Geometry check sheet. Reference: the model listing, model coordinates, mm. A direction names the side the tool comes from. Give positions to 0.01 mm unless a question says otherwise; leave off trailing zeros. Loops run counter-clockwise (first coordinate to the right, second up) from the corner with the lowest first, then second, coordinate; pieces in that order, holes last. Notation, with made-up numbers: (18, -21) -> (37, -21) arc R30 ccw to (37, 8) -> close; hole circle Ø9 at (-37.75, 49). An arc over 180 degrees is marked (long way). Write each question's results on one line, items separated by ' | '. Start each with the question number.
1) Sectioned sample at C-C on z = -4.15. Record the cut outline in (x, y).
2) Sectioned sample at A-A on y = 0. Record the cut outline in (x, z).
3) Scan lines: line 1 (Y direction, x = 0, z = -1.9); line 2 (Z direction, x = 5, y = 0.5); line 3 (Y direction, x = -2, z = -2.35). Record each from-to range of solid material in increasing order. Write a range as from..to.
4) Set-up check for faces 1 (the face through (5.96, -1.88, -0.51)), 2 (the face through (-1, 5, -1)): record each of +Z, -Z, +X, -X, +Y, -Y from which the full face is reachable in a straight line by a thin tool's end or side.
5) Depth check by flat-ended pin: pin 1 (2 mm diameter, centred on x = 2.5, z = -5, fed in from -Y); pin 2 (3 mm diameter, centred on y = 4, z = -1.5, fed in from -X); pin 3 (5.5 mm diameter, centred on x = 0, y = 0, fed in from +Z). Enter the tip coordinate at first touch or a pass-through.
6) Sectioned sample at D-D on x = 5.75. Record the cut outline in (y, z).
```python
from build123d import *


# Read off the part's stored shape, not the designer's step: Оболочка1
with BuildPart() as part:
    # Эскиз1 → Повернуть1 (revolve)
    with BuildSketch(Plane(origin=(0, 0, 0), x_dir=(1, 0, 0), z_dir=(0, 1, 0))):
        with BuildLine():
            Line((0, 6), (0, 1))
            Line((0, 1), (3.872983346, 1))
            ThreePointArc((3.872983346, 1), (3.968118785, 1.49598283), (4, 2))
            ThreePointArc((4, 2), (2.828427125, 4.828427125), (0, 6))
        make_face()
        with BuildLine():
            Line((3.872983346, 1), (0, 1))
            Line((0, 1), (0, 0))
            Line((0, 0), (3.464101615, 0))
            ThreePointArc((3.464101615, 0), (3.702459174, 0.486132084), (3.872983346, 1))
        make_face()
        with BuildLine():
            ThreePointArc((4, 2), (3.968118785, 1.49598283), (3.872983346, 1))
            ThreePointArc((3.872983346, 1), (3.702459174, 0.486132084), (3.464101615, 0))
            Line((3.464101615, 0), (6.25, 0))
            Line((6.25, 0), (6.25, 1))
            Line((6.25, 1), (4.8, 1))
            ThreePointArc((4.8, 1), (4.234314575, 1.234314575), (4, 1.8))
            Line((4, 1.8), (4, 2))
        make_face()
    revolve(axis=Axis((0, 0, -1), (0, 0, -1)))

    # Оболочка1 outline → Оболочка1 (revolve, cut)
    with BuildSketch(Plane.XZ):
        with BuildLine():
            ThreePointArc((3, -1.8), (3.527207794, -0.527207794), (4.8, 0))
            Line((4.8, 0), (0, 0))
            Line((0, 0), (0, -5))
            ThreePointArc((0, -5), (2.121320345, -4.121320342), (3, -1.999999997))
            Line((3, -1.999999997), (3, -1.8))
        make_face()
    revolve(axis=Axis((0, 0, 0), (0, 0, 1)), mode=Mode.SUBTRACT)


solid = part.part
```
Result:
1) outline: circle Ø6.75 at (0, 0); hole circle Ø4.18 at (0, 0)
2) outline: (-6.25, -1) -> (-4.8, -1) arc R0.8 cw to (-4, -1.8) -> (-4, -2) arc R4 ccw to (4, -2) -> (4, -1.8) arc R0.8 cw to (4.8, -1) -> (6.25, -1) -> (6.25, 0) -> (4.8, 0) arc R1.8 ccw to (3, -1.8) -> (3, -2) arc R3 cw to (-3, -2) -> (-3, -1.8) arc R1.8 ccw to (-4.8, 0) -> (-6.25, 0) -> close
3) line 1: -4..-3, 3..4 | line 2: -1..0 | line 3: -3.45..-2.21, 2.21..3.45
4) face 1: +Z, -Z | face 2: -Z
5) pin 1: y = -2.75 | pin 2: x = -5.69 | pin 3: z = -3.2
6) outline: (-2.45, -1) -> (2.45, -1) -> (2.45, 0) -> (-2.45, 0) -> close
